```python
from build123d import *

# Parameters (mm, degrees)
SKETCH2_R          = 8.1
CUT_EXTRUDE1_DEPTH = 6
SKETCH3_R          = 7
CUT_EXTRUDE2_DEPTH = 6


with BuildPart() as part:
    # Sketch1 → Revolve1 (revolve)
    with BuildSketch(Plane.XY, mode=Mode.PRIVATE) as revolve1_sk:
        Polygon((2.5, 8), (15, 8), (15, 4.4), (14.6, 4), (15, 3.6), (15, 0), (2.5, 0), align=None)
    revolve(revolve1_sk.sketch.rotate(Axis((0, 0, 0), (0, 1, 0)), 90), axis=Axis((0, 0, 0), (0, 1, 0)))

    # Sketch2 → Cut-Extrude1 (cut)
    with BuildSketch(Plane(origin=(0, 8, 0), x_dir=(1, 0, 0), z_dir=(0, 1, 0))):
        with Locations(Location((0, 0, 0), (0, 0, 270))):
            Circle(SKETCH2_R)
    extrude(amount=-CUT_EXTRUDE1_DEPTH, mode=Mode.SUBTRACT)

    # Sketch3 → Cut-Extrude2 (cut)
    with BuildSketch(Plane(origin=(0, 2, 0), x_dir=(1, 0, 0), z_dir=(0, 1, 0))):
        with Locations(Location((0, 0, 0), (0, 0, 270))):
            Circle(SKETCH3_R)
    extrude(amount=-CUT_EXTRUDE2_DEPTH, mode=Mode.SUBTRACT)


solid = part.part
```
Can you work these out from the model? Positions are in its coordinate system, mm. A direction names the side the tool comes from. Coordinates: 2 decimals unless noted, no trailing zeros. Order: outer loops, then holes, each group sorted by start corner. A loop starts at its lowest first (then second) coordinate and runs counter-clockwise, first axis right, second up.
1. If we section it at D-D (y = 0.75): Please give me the cut outline in (x, z).
2. For faces 1 (the face through (6, 8, 6)), 2 (the face through (-7.186, 5.042, 3.738)), which set-ups out of +Z, -Z, +X, -X, +Y, -Y let a thin tool reach every point of the face, with its end or its side?
3. If we section it at C-C (y = 7.5): Please give me the cut outline in (x, z), then the cut area to 3 significant figures.
4. If we section it at A-A (x = 0): Please give me the cut outline in (y, z), then the cut area to 3 significant figures.
5. I need wall thicknesses on line 1 (X direction, y = 5, z = 0); line 2 (X direction, y = 0.85, z = 0). Which ranges of each line are inside material? Lowest first, please.
6. I'm going to push flat-ended pins straight in: pin 1 (3 mm diameter, centred on x = -5.5, y = 4, fed in from +Z); pin 2 (8 mm diameter, centred on x = 3.5, z = -1, fed in from +Y); pin 3 (1 mm diameter, centred on y = 6, z = -7.5, fed in from +X). Where does each tip first touch, or does it pass through?
7. If we section it at B-B (z = 0): Please give me the cut outline in (x, y).
Entries:
1. outline: circle Ø30 at (0, 0); hole circle Ø14 at (0, 0)
2. face 1: +Z, -Z, +X, -X, +Y
2. face 2: +Y
3. outline: circle Ø30 at (0, 0); hole circle Ø16.2 at (0, 0)
3. area: 501 mm2
4. outline: (0, -15) - (3.6, -15) - (4, -14.6) - (4.4, -15) - (8, -15) - (8, -8.1) - (2, -8.1) - (2, -7) - (0, -7) - close; (0, 7) - (2, 7) - (2, 8.1) - (8, 8.1) - (8, 15) - (4.4, 15) - (4, 14.6) - (3.6, 15) - (0, 15) - close
4. area: 114 mm2
5. line 1: x = -15 to -8.1, 8.1 to 15
5. line 2: x = -15 to -7, 7 to 15
6. pin 1: stops at z = 14.44
6. pin 2: stops at y = 2
6. pin 3: stops at x = 13.27
7. outline: (-15, 0) - (-7, 0) - (-7, 2) - (-8.1, 2) - (-8.1, 8) - (-15, 8) - (-15, 4.4) - (-14.6, 4) - (-15, 3.6) - close; (7, 0) - (15, 0) - (15, 3.6) - (14.6, 4) - (15, 4.4) - (15, 8) - (8.1, 8) - (8.1, 2) - (7, 2) - close
